```python
from build123d import *

# Parameters (mm, degrees)
CYLINDER037_R     = 3
CYLINDER037_DEPTH = 10
CYLINDER036_R     = 5
CYLINDER036_DEPTH = 4
CYLINDER035_R     = 0.5
CYLINDER035_DEPTH = 10
CYLINDER034_R     = 2.5
CYLINDER034_DEPTH = 10
BOX012_W          = 4
BOX012_H          = 10
BOX012_DEPTH      = 5
CYLINDER033_R     = 5
CYLINDER033_DEPTH = 10


with BuildPart() as cylinder037:
    # Cylinder037 → Cylinder037 (new body)
    with BuildSketch(Plane(origin=(18, 0, -6), x_dir=(1, 0, 0), z_dir=(0, 0, 1))):
        Circle(CYLINDER037_R)
    extrude(amount=CYLINDER037_DEPTH)


with BuildPart() as cut031:
    # Cylinder036 → Cylinder036 (new body)
    with BuildSketch(Plane(origin=(18, 0, -4), x_dir=(1, 0, 0), z_dir=(0, 0, 1))):
        Circle(CYLINDER036_R)
    extrude(amount=CYLINDER036_DEPTH)

    # Cut031: cut Cylinder037
    add(cylinder037.part, mode=Mode.SUBTRACT)


with BuildPart() as cut031_1:
    # Cut031 placement: moved
    add(cut031.part.moved(Location((-18, 0, 0))))


with BuildPart() as sphere008:
    # Sphere008 → Sphere008 (revolve)
    with BuildSketch(Plane(origin=(0, 0, -5), x_dir=(1, 0, 0), z_dir=(0, -1, 0))):
        with BuildLine():
            ThreePointArc((0, -6), (6, 0), (0, 6))
            Line((0, 6), (0, -6))
        make_face()
    revolve(axis=Axis((0, 0, -5), (0, 0, 1)))


with BuildPart() as cylinder035:
    # Cylinder035 → Cylinder035 (new body)
    with BuildSketch(Plane(origin=(5, 0, -7), x_dir=(0, 0, 1), z_dir=(-1, 0, 0))):
        Circle(CYLINDER035_R)
    extrude(amount=CYLINDER035_DEPTH)


with BuildPart() as cylinder034:
    # Cylinder034 → Cylinder034 (new body)
    with BuildSketch(Plane.XY.offset(-10)):
        Circle(CYLINDER034_R)
    extrude(amount=CYLINDER034_DEPTH)


with BuildPart() as cube012:
    # Box012 → Box012 (new body)
    with BuildSketch(Plane(origin=(-2, -5, -10), x_dir=(1, 0, 0), z_dir=(0, 0, 1))):
        with Locations((2, 5)):
            Rectangle(BOX012_W, BOX012_H)
    extrude(amount=BOX012_DEPTH)


with BuildPart() as fusion005011:
    # Cylinder033 → Cylinder033 (new body)
    with BuildSketch(Plane.XY.offset(-10)):
        Circle(CYLINDER033_R)
    extrude(amount=CYLINDER033_DEPTH)

    # Cut028: cut Cube012
    add(cube012.part, mode=Mode.SUBTRACT)

    # Cut029: cut Cylinder034
    add(cylinder034.part, mode=Mode.SUBTRACT)

    # Cut030: cut Cylinder035
    add(cylinder035.part, mode=Mode.SUBTRACT)

    # Common006: intersect Sphere008
    add(sphere008.part, mode=Mode.INTERSECT)

    # Fusion005010: union Cut031
    add(cut031_1.part)


with BuildPart() as fusion005011_1:
    # Fusion005011 placement: moved
    add(fusion005011.part.moved(Location((0, 0, -37))))


solid = fusion005011_1.part
```
Source: CAD feature listing. Evaluate the final solid. Frame: model axes, mm. A direction names the side the tool comes from. Give positions to 0.01 mm unless a question says otherwise; leave off trailing zeros. Loops run counter-clockwise (first coordinate to the right, second up) from the corner with the lowest first, then second, coordinate; pieces in that order, holes last. Notation, with made-up numbers: (12.5, 40) -> (71.5, 40) arc R23 ccw to (71.5, 65) -> close; hole circle Ø2 at (78, 37). An arc over 180 degrees is marked (long way). Put each result on its own line as item: value. Start each with the question number.
1) Cut plane B-B (x = 0). Return loops of the section in (y, z), then the cut area to 3 significant figures.
2) Contact query for flat-ended pins moving along their axis: P1, Ø2.5, axis at y = -3, z = -45, coming from the -X side; P2, Ø3.5, axis at y = -3.5, z = -44, coming from the +X side; P3, Ø1.8, axis at x = 0.5, y = -2.5, coming from the -Z side. Output: stop coordinate, or through.
3) Reachability of faces 1 (the face through (-3, 0, -47)), 2 (the face through (-2, 3, -45)) from +Z, -Z, +X, -X, +Y, -Y: full face, straight path, thin tool, end or side. Return the list, or none.
4) Draft query along X for faces 3 (the face through (2, 3, -45)), 4 (the face through (4.619, -1.915, -41.217)), 5 (the face through (3.7, 0, -44.5)). Return one class per face: released by +X, released by -X, zero draft, split by the parting line, or undercut.
5) Material intervals for probe 1 along Y at (x, z) = (2, -41.25); probe 2 along Z at (x, y) = (-1.75, -3.75); probe 3 along Z at (x, y) = (4.05, 0), sorted ascending.
6) Cut plane C-C (z = -43.25). Return loops of the section in (x, y), then the cut area to 3 significant figures.
7) Cut plane A-A (y = 0). Return loops of the section in (x, z), then the cut area to 3 significant figures.
8) Cut plane D-D (y = -1.25). Return loops of the section in (x, z).
Results are:
1. outline: (-5, -42) -> (-2.5, -42) -> (-2.5, -37) -> (-5, -37) -> close; (2.5, -42) -> (5, -42) -> (5, -37) -> (2.5, -37) -> close
1. area: 25.0 mm2
2. P1: stops at x = -4.68
2. P2: stops at x = 4.68
2. P3: stops at z = -42
3. face 1: -Z, +X, -X, +Y, -Y
3. face 2: -Z, +Y, -Y
4. face 3: undercut
4. face 4: split by the parting line
4. face 5: zero draft
5. probe 1: y = -4.58 to -1.5, 1.5 to 4.58
5. probe 2: z = -42 to -37
5. probe 3: z = -46.43 to -44.5, -43.5 to -37
6. outline: (-2, -4.58) -> (-2, -1.5) arc R2.5 cw to (-2, 1.5) -> (-2, 4.58) arc R5 ccw to start; (2, -4.58) arc R5 ccw to (2, 4.58) -> (2, 1.5) arc R2.5 cw to (2, -1.5) -> close
6. area: 37.6 mm2
7. outline: (-5, -45.32) arc R6 ccw to (-3.32, -47) -> (-2.5, -47) -> (-2.5, -44.5) -> (-5, -44.5) -> close; (-5, -43.5) -> (-2.5, -43.5) -> (-2.5, -37) -> (-5, -37) -> close; (2.5, -47) -> (3.32, -47) arc R6 ccw to (5, -45.32) -> (5, -44.5) -> (2.5, -44.5) -> close; (2.5, -43.5) -> (5, -43.5) -> (5, -37) -> (2.5, -37) -> close
7. area: 42.5 mm2
8. outline: (-4.84, -45.32) arc R5.87 ccw to (-3.07, -47) -> (-2.17, -47) -> (-2.17, -37) -> (-4.84, -37) -> close; (2.17, -47) -> (3.07, -47) arc R5.87 ccw to (4.84, -45.32) -> (4.84, -37) -> (2.17, -37) -> close
